The listing builds one solid part. Answer for the finished solid, in the listing's coordinates (mm). Face numbers are marked on the shaded views. A direction names the side the tool comes from. Coordinates: 2 decimals unless noted, no trailing zeros. Order: outer loops, then holes, each group sorted by start corner. A loop starts at its lowest first (then second) coordinate and runs counter-clockwise, first axis right, second up. Notation, with made-up numbers: (35, 21) - (57, 21) arc R22 cw to (57, 58) - close; hole circle Ø8 at (11.5, 17). An arc over 180 degrees is marked (long way). Use a Markdown table: item, result. Add a question column.
Item 1: The part is cut by section C-C, the plane y = -2.75. Give the vertices of the cut face in (x, z).
Item 2: Flat-ended cylindrical pins translate along their axes: P1, Ø3.5, axis at y = 6.5, z = -13, coming from the -X side; P2, Ø2.5, axis at y = -3.5, z = -11.5, coming from the -X side; P3, Ø1, axis at y = 1.5, z = -20, coming from the -X side; P4, Ø1.8, axis at x = -2.5, y = -1.5, coming from the +Z side. Find the tip coordinate at first contact, or state that the pin passes through.
Item 3: Find the intervals of material crossed by line 1 along Z through (x, y) = (-8.5, 3.25); line 2 along X through (y, z) = (11.75, -25); line 3 along Z through (x, y) = (-2.75, 4.25), in increasing order.
Item 4: The mould has two halves that part along Z. Classify the marked faces 1, 2, 3 and 4: released by +Z, released by -Z, zero draft, split by the parting line, or undercut.
Item 5: The part is cut by section A-A, the plane z = -18.5. Give the vertices of the cut face in (x, y).
Item 6: The part is cut by section D-D, the plane z = -10.5. Give the vertices of the cut face in (x, y).
Item 7: The part is cut by section B-B, the plane x = -4. Give the vertices of the cut face in (y, z).
Item 8: For the marked faces 5, 6, 7 and 8, determine the directions among +Z, -Z, +X, -X, +Y, -Y from which every point of the face is accessible in a straight line to the end or side of a thin tool.
Autodesk Inventor part; units mm, degrees
ref_plane "YZ Plane" through (0, 0, 0) normal (1, 0, 0) x (0, 1, 0)
ref_plane "XZ Plane" through (0, 0, 0) normal (0, 1, 0) x (-1, 0, 0)
ref_plane "XY Plane" through (0, 0, 0) normal (0, 0, 1) x (1, 0, 0)
sketch "スケッチ1" plane through (0, 0, 0) normal (0, 1, 0) x (-1, 0, 0)
  line L0 (10, -0.3) -> (0, -0.3)
  line L1 (0, -0.3) -> (0, -5)
  line L2 (0, -5) -> (10, -5)
  line L3 (10, -5) -> (10, -0.3)
  line L4 (8.5, -5) -> (0, -5)
  line L5 (0, -5) -> (0, -18)
  line L6 (0, -18) -> (8.5, -18)
  line L7 (8.5, -18) -> (8.5, -5)
  line L8 (10, -18) -> (0, -18)
  line L9 (0, -18) -> (0, -22.7)
  line L10 (0, -22.7) -> (10, -22.7)
  line L11 (10, -22.7) -> (10, -18)
  point P0 (0, 0)
  dimension "d0" = 10
  dimension "d2" = 1.5
  dimension "d3" = 13
  dimension "d34" = 5
  dimension "d35" = 0.3
extrude "押し出し1" add sketch "スケッチ1" along normal blind 15
sketch "スケッチ3" plane through (-10, 0, -18) normal (0, 0, 1) x (1, 0, 0)
  line L0 (0, 0) -> (1.5, 0)
  line L1 (1.5, 0) -> (1.5, 15)
  line L2 (0, 15) -> (1.5, 15)
  line L3 (0, 0) -> (0, 15)
  line L4 (0, 0) -> (10, 0)
  line L5 (10, 0) -> (10, 15)
  line L6 (0, 15) -> (10, 15)
  line L7 (0, 0) -> (0, 15)
  circle A0 centre (4.5, 12) radius 3
  circle A1 centre (4.5, 12) radius 2.5
  line L8 (2, 12) -> (2, 0)
  line L9 (4.5, 14.5) -> (10, 14.5)
  point P0 (1.5, 15)
  point P1 (1.5, 0)
  dimension "d6" = 6
  dimension "d7" = 0.5
extrude "押し出し2" cut sketch "スケッチ3" along normal up to surface (13 mm away) contours L1 A0 L8 L4 | L1 L6 A0 | A0 L9 A1 L8 | L6 L5 L9 A0 picked at (5.4334, 14.5914)
sketch "スケッチ4" plane through (0, 15, 0) normal (0, 1, 0) x (1, 0, 0)
  line L0 (0, 5) -> (-10, 5)
  line L1 (-10, 5) -> (-10, 0.3)
  line L2 (-10, 0.3) -> (0, 0.3)
  line L3 (0, 0.3) -> (0, 5)
  point P0 (0, 0)
extrude "押し出し3" cut sketch "スケッチ4" against normal up to surface (0.5 mm away)
sketch "スケッチ5" plane through (-8, 0, -18) normal (-1, 0, 0) x (0, 0, 1)
  line L0 (13, 0) -> (18, 0)
  line L1 (13, 0) -> (3, 0)
  line L2 (3, 0) -> (3, 15)
  line L3 (3, 15) -> (13, 15)
  line L4 (13, 15) -> (13, 0)
  line L5 (6, 12) -> (10, 12)
  line L6 (10, 12) -> (10, 2)
  line L7 (10, 2) -> (6, 2)
  line L8 (6, 2) -> (6, 12)
  line L9 (13, 0) -> (0, 0)
  point P0 (6.5, 0)
  point P1 (8, 12)
  point P2 (8, 15)
  dimension "d12" = 10
  dimension "d13" = 3
  dimension "d14" = 2
  dimension "d15" = 4
  dimension "d21" = 15
extrude "押し出し4" add sketch "スケッチ5" along normal blind 2 contours L5 L6 L7 L8
sketch "スケッチ6" plane through (-8, 2, -8) normal (0, 0, 1) x (1, 0, 0)
  line L0 (0, 10) -> (0, 0)
  line L1 (0, 10) -> (-2, 10)
  line L2 (-2, 0) -> (-2, 10)
  line L3 (0, 0) -> (-2, 0)
  line L4 (0, 0) -> (0, 10)
  arc A0 (0, 9.5) -> (-2, 0.5) centre (19.25, 0.5) ccw
  line L5 (-2, 0.5) -> (0, 0.5)
  point P0 (8, -2)
  point P1 (0, 0.5)
  dimension "d22" = 0.5
  dimension "d23" = 0.5
extrude "押し出し5" cut sketch "スケッチ6" against normal up to surface (4 mm away) contours L0 A0 L2 L1 | L0 L3 L2 L5
fillet "フィレット1" radius 0.5 2 edges at (-9.494, 7.1098, -12) (-9.494, 7.1098, -8)
mirror "ミラー1" about plane through (0, 0, -0.3) normal (1, 0, 0)
sketch "スケッチ7" plane through (-5.5, 14.5, -5) normal (0, 0, -1) x (-1, 0, 0)
  line L0 (4.5, 0) -> (0, 0)
  arc A0 (2.5, -2.5) -> (0, 0) centre (0, -2.5) ccw
  line L1 (2.5, -14.5) -> (2.5, -2.5)
  line L2 (4.5, -14.5) -> (2.5, -14.5)
  line L3 (4.5, -14.5) -> (4.5, 0)
  line L4 (-15.5, 0) -> (-11, 0)
  line L5 (-15.5, -14.5) -> (-15.5, 0)
  line L6 (-15.5, -14.5) -> (-13.5, -14.5)
  line L7 (-13.5, -14.5) -> (-13.5, -2.5)
  arc A1 (-11, 0) -> (-13.5, -2.5) centre (-11, -2.5) ccw
  point P0 (-5.5, -14.5)
extrude "押し出し6" cut sketch "スケッチ7" against normal blind 0.5
sketch "スケッチ13" plane through (-10, 14.5, -0.3) normal (0, 1, 0) x (1, 0, 0)
  arc A0 (21.586, 79.673) -> (5.1529, 40) centre (157.8276, 0) ccw
  arc A1 (46.2266, 111.6009) -> (0, 0) centre (157.8276, 0) ccw
  line L0 (0, 22.4) -> (0, 32.4)
  line L1 (0, 22.4) -> (0, 22.4)
  line L2 (0, 17.7) -> (0, 22.4)
  line L3 (0, 17.7) -> (2, 17.7)
  line L4 (0, 32.4) -> (20, 32.4)
  point P0 (10, -0.3)
  point P1 (0.9956, 17.7)
  point P2 (3.3615, 32.4)
extrude "押し出し14" cut sketch "スケッチ13" along normal through all both and the other way through all
mirror "ミラー2" about plane through (0, 0, 0) normal (1, 0, 0) of "押し出し14"
sketch "スケッチ14" plane through (0, 0, 0) normal (0, -1, 0) x (1, 0, 0)
  line L0 (1.5, -6) -> (-1.5, -6)
  line L1 (-1.5, -6) -> (-1.5, -16)
  line L2 (-1.5, -16) -> (1.5, -16)
  line L3 (1.5, -16) -> (1.5, -6)
  line L4 (5, -9.5) -> (-5, -9.5)
  line L5 (-5, -9.5) -> (-5, -12.5)
  line L6 (-5, -12.5) -> (5, -12.5)
  line L7 (5, -12.5) -> (5, -9.5)
  point P0 (0, 0)
  point P1 (5, -11)
  point P2 (1.5, -11)
  point P3 (0, -6)
  point P4 (0, -9.5)
  point P5 (1.5, -9.5)
  point P6 (-1.5, -9.5)
  point P7 (-1.5, -12.5)
  point P8 (1.5, -12.5)
  dimension "d65" = 10
  dimension "d66" = 3
  dimension "d70" = 6
extrude "押し出し15" add sketch "スケッチ14" along normal blind 5
sketch "スケッチ15" plane through (0, 0, 0) normal (0, -1, 0) x (1, 0, 0)
  arc A0 (-9.0044, -18) -> (-8.4023, -22.7) centre (147.8276, -0.3) ccw
  line L0 (-9.0044, -18) -> (9.0044, -18)
  line L1 (9.0044, -18) -> (9.0044, -22.7)
  line L2 (9.0044, -22.7) -> (-9.0044, -22.7)
  line L3 (-9.0044, -22.7) -> (-9.0044, -18)
  point P0 (0, 0)
  point P1 (8.4023, -22.7)
extrude "押し出し16" cut sketch "スケッチ15" against normal through all
sketch "スケッチ16" plane through (5.5, 14.5, -18) normal (0, 0, -1) x (-1, 0, 0)
  line L0 (13.5, -14.5) -> (13.5, -2.5)
  arc A0 (13.5, -2.5) -> (11, 0) centre (11, -2.5) ccw
  line L1 (11, 0) -> (0, 0)
  arc A1 (0, 0) -> (-2.5, -2.5) centre (0, -2.5) ccw
  line L2 (-2.5, -14.5) -> (-2.5, -2.5)
  line L3 (13.5, -14.5) -> (-2.5, -14.5)
  line L4 (6.75, -14.5) -> (4.25, -14.5)
  line L5 (4.25, -14.5) -> (4.25, 0)
  line L6 (4.25, 0) -> (6.75, 0)
  line L7 (6.75, 0) -> (6.75, -14.5)
  point P0 (5.5, -14.5)
  point P1 (5.5, -14.5)
  point P2 (6.75, 0)
  dimension "d73" = 2.5
extrude "押し出し17" add sketch "スケッチ16" along normal blind 15 contours L3 L7 L1 A0 L0 | L3 L2 A1 L1 L5
sketch "スケッチ17" plane through (5.5, 14.5, -33) normal (0, 0, -1) x (-1, 0, 0)
  line L0 (13.5, -14.5) -> (-2.5, -14.5)
  line L1 (-2.5, -14.5) -> (-2.5, -8.5)
  line L2 (-2.5, -8.5) -> (13.5, -8.5)
  line L3 (13.5, -8.5) -> (13.5, -14.5)
  line L4 (-2.5, -2.5) -> (-2.5, -14.5)
  point P0 (5.5, -14.5)
  dimension "d76" = 6
extrude "押し出し18" cut sketch "スケッチ17" against normal blind 15
equation "\"d22\" = d23"
properties part number "connector_male"
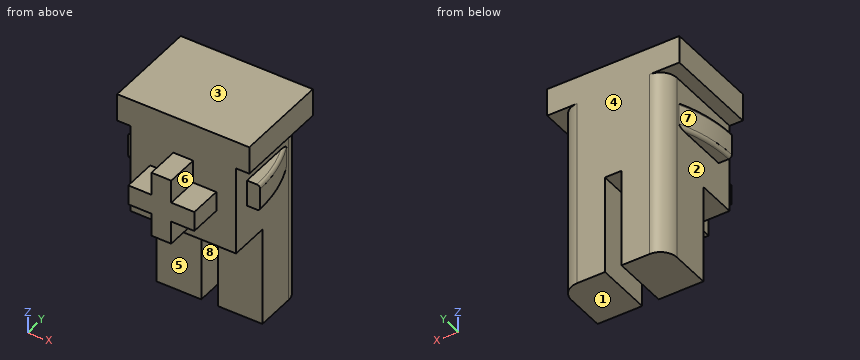
Solution:
| question | item | result |
|---|---|---|
| 1 | outline | (-5, -12.5) - (-1.5, -12.5) - (-1.5, -16) - (1.5, -16) - (1.5, -12.5) - (5, -12.5) - (5, -9.5) - (1.5, -9.5) - (1.5, -6) - (-1.5, -6) - (-1.5, -9.5) - (-5, -9.5) - close |
| 2 | P1 | stops at x = -9.78 |
| 2 | P2 | stops at x = -5 |
| 2 | P3 | passes through |
| 2 | P4 | stops at z = -9.5 |
| 3 | line 1 | z = -12 to -8, -4.5 to -0.3 |
| 3 | line 2 | x = -8 to -1.25, 1.25 to 8 |
| 3 | line 3 | z = -18 to -0.3 |
| 4 | face 1 | released by -Z |
| 4 | face 2 | undercut |
| 4 | face 3 | released by +Z |
| 4 | face 4 | zero draft |
| 5 | outline | (-8, 6) - (-1.25, 6) - (-1.25, 14.5) - (-5.5, 14.5) arc R2.5 ccw to (-8, 12) - close; (1.25, 6) - (8, 6) - (8, 12) arc R2.5 ccw to (5.5, 14.5) - (1.25, 14.5) - close |
| 6 | outline | (-10, 2.5) - (-8, 2.5) - (-8, 0) - (-5, 0) - (-5, -5) - (5, -5) - (5, 0) - (8, 0) - (8, 2.5) - (10, 2.5) arc R21.25 ccw to (8, 11.5) - (8, 12) arc R2.5 ccw to (5.5, 14.5) - (-5.5, 14.5) arc R2.5 ccw to (-8, 12) - (-8, 11.5) arc R21.25 ccw to start |
| 7 | outline | (-5, -12.5) - (0, -12.5) - (0, -18) - (6, -18) - (6, -33) - (14.5, -33) - (14.5, -0.3) - (0, -0.3) - (0, -9.5) - (-5, -9.5) - close |
| 8 | face 5 | -Z, +X, -X, -Y |
| 8 | face 6 | +Z, +X, -Y |
| 8 | face 7 | -Z, -X, +Y |
| 8 | face 8 | -Z, +Y, -Y |
